Here's the drawing with two shaded views (mm, measured from the low corner). I have some questions. A direction names the side the tool comes from. Round coordinates to 2 decimals unless told otherwise and drop trailing zeros. Write each loop counter-clockwise with the first axis right and the second up, starting at its lowest first coordinate (ties: lowest second). Pieces come first, ordered by that corner, then holes. Notation, with made-up numbers: (62.25, 84.5) -> (112.25, 84.5) arc R23 ccw to (112.25, 110.5) -> close; hole circle Ø10 at (44, 38). An arc over 180 degrees is marked (long way). Use CSV: the item, a comma, the result in double quotes.
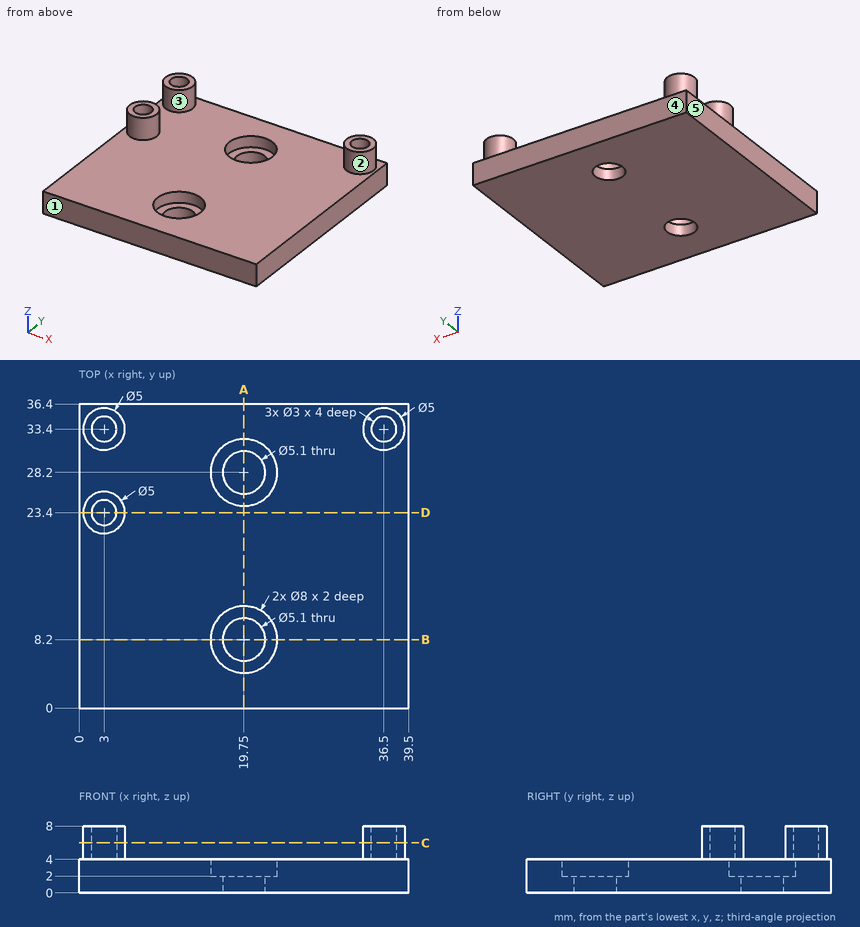
Q1. Suppose I cut it at C-C (z = 6). Write out the boundary of the cut face in (x, y).
Resolved:
outline,"circle Ø5 at (3, 23.4); circle Ø5 at (3, 33.4); circle Ø5 at (36.5, 33.4); hole circle Ø3 at (3, 23.4); hole circle Ø3 at (3, 33.4); hole circle Ø3 at (36.5, 33.4)"
Q2. Suppose I cut it at A-A (x = 19.75). Write out the boundary of the cut face in (y, z), and give its area (3 significant figures).
Resolved:
outline,"(0, 0) -> (5.65, 0) -> (5.65, 2) -> (4.2, 2) -> (4.2, 4) -> (0, 4) -> close; (10.75, 0) -> (25.65, 0) -> (25.65, 2) -> (24.2, 2) -> (24.2, 4) -> (12.2, 4) -> (12.2, 2) -> (10.75, 2) -> close; (30.75, 0) -> (36.4, 0) -> (36.4, 4) -> (32.2, 4) -> (32.2, 2) -> (30.75, 2) -> close"
area,"93.2 mm^2"
Q3. Please list where these lines run through material, in increasing order: probe 1 along Y at (x, z) = (3, 5.2); probe 2 along X at (y, z) = (33.4, 6.95); probe 3 along Y at (x, z) = (19.75, 2.6).
Resolved:
probe 1,"y = 20.9 to 21.9, 24.9 to 25.9, 30.9 to 31.9, 34.9 to 35.9"
probe 2,"x = 0.5 to 1.5, 4.5 to 5.5, 34 to 35, 38 to 39"
probe 3,"y = 0 to 4.2, 12.2 to 24.2, 32.2 to 36.4"
Q4. Suppose I cut it at D-D (y = 23.4). Write out the boundary of the cut face in (x, z).
Resolved:
outline,"(0, 0) -> (39.5, 0) -> (39.5, 4) -> (5.5, 4) -> (5.5, 8) -> (4.5, 8) -> (4.5, 4) -> (1.5, 4) -> (1.5, 8) -> (0.5, 8) -> (0.5, 4) -> (0, 4) -> close"
Q5. On a 3-axis mill with a long thin cutter (end or side, diameter ignored), from which of +Z, -Z, +X, -X, +Y, -Y can I reach the whole of each face in a straight line? I mean the marked faces 1 and 2. Say none if no direction works.
Resolved:
face 1,"+Z, -Z, +X, -X, -Y"
face 2,"+Z"
Q6. If we mould it in two halves opening along X, with no side actions, what happens to the marked faces 3, 4 and 5? For each: released by +X, released by -X, zero draft, split by the parting line, or undercut.
Resolved:
face 3,"undercut"
face 4,"zero draft"
face 5,"released by -X"
Q7. Suppose I cut it at B-B (y = 8.2). Write out the boundary of the cut face in (x, z), and give its area (3 significant figures).
Resolved:
outline,"(0, 0) -> (17.2, 0) -> (17.2, 2) -> (15.75, 2) -> (15.75, 4) -> (0, 4) -> close; (22.3, 0) -> (39.5, 0) -> (39.5, 4) -> (23.75, 4) -> (23.75, 2) -> (22.3, 2) -> close"
area,"132 mm^2"
Q8. Will these pins go through, and if not, where does the flat tip stop? P1, Ø1.5, axis at x = 3, y = 22.5, coming from the +Z side; P2, Ø10, axis at x = 26.5, y = 10, coming from the +Z side; P3, Ø4, axis at x = 19, y = 26.5, coming from the +Z side.
Resolved:
P1,"stops at z = 8"
P2,"stops at z = 4"
P3,"stops at z = 2"
